Work out the finished part from the listing and answer in its coordinate system (mm). Round coordinates to 2 decimals unless told otherwise and drop trailing zeros. Write each loop counter-clockwise with the first axis right and the second up, starting at its lowest first coordinate (ties: lowest second). Pieces come first, ordered by that corner, then holes. Notation, with made-up numbers: M -33,58 L -20,58 A19 cw -20,62 Z; hole C 59.25,39 d3. An arc over 180 degrees is marked long. One line per item, written item: value. Start each with the question number.
Q1. Find section A-A (y = -73.5). Write down the section's boundary in (x, z).
Q2. Find section D-D (y = 1). Write down the section's boundary in (x, z), and give its area (3 significant figures).
Q3. Find section C-C (z = 2.4). Write down the section's boundary in (x, y).
Q4. Consider probe 1 along Y at (x, z) = (0, 1.05); probe 2 along Y at (x, z) = (-1.5, 2.65); probe 3 along X at (y, z) = (-76, 1.15). Determine where each line is inside the solid, lowest interval first.
Q5. Find section B-B (x = 0). Write down the section's boundary in (y, z).
Q6. Given pin 1 Ø4 at (x, y) = (7.5, -20.5) entering from -Z, flat-ended and moving along its own axis, determine where the tip first touches the part or whether it passes through.
from build123d import *

# Parameters (mm, degrees)
SKETCH1_R           = 2.5
BOSS_EXTRUDE1_DEPTH = 3


with BuildPart() as part:
    # Sketch1 → Boss-Extrude1 (new body)
    with BuildSketch(Plane.XY):
        with BuildLine():
            Line((10, 0), (10, -100))
            Line((10, -100), (-10, -100))
            Line((-10, -100), (-10, 0))
            ThreePointArc((-10, 0), (0, 10), (10, 0))
        make_face()
        Circle(SKETCH1_R, mode=Mode.SUBTRACT)
        with BuildLine():
            Line((5, -20), (5, -40))
            ThreePointArc((5, -40), (0, -45), (-5, -40))
            Line((-5, -40), (-5, -20))
            ThreePointArc((-5, -20), (0, -15), (5, -20))
        make_face(mode=Mode.SUBTRACT)
        with BuildLine():
            Line((-5, -85), (-5, -65))
            ThreePointArc((-5, -65), (0, -60), (5, -65))
            Line((5, -65), (5, -85))
            ThreePointArc((5, -85), (0, -90), (-5, -85))
        make_face(mode=Mode.SUBTRACT)
    extrude(amount=BOSS_EXTRUDE1_DEPTH)


solid = part.part
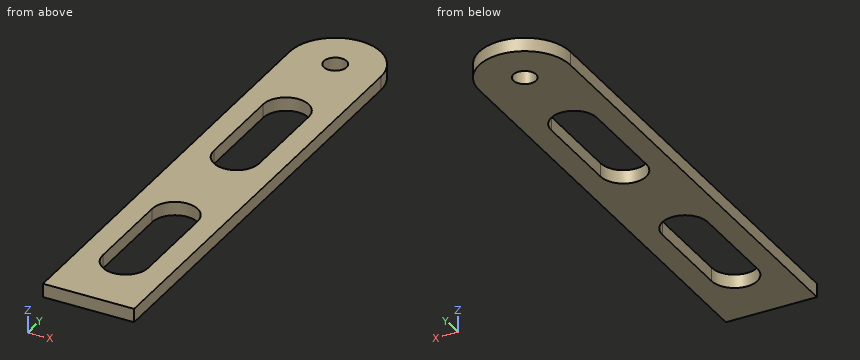
The answers:
1. outline: M -10,0 L -5,0 L -5,3 L -10,3 Z; M 5,0 L 10,0 L 10,3 L 5,3 Z
2. outline: M -9.95,0 L -2.29,0 L -2.29,3 L -9.95,3 Z; M 2.29,0 L 9.95,0 L 9.95,3 L 2.29,3 Z
2. area: 46.0 mm2
3. outline: M -10,-100 L 10,-100 L 10,0 A10 ccw -10,0 Z; hole M -5,-85 A5 ccw 5,-85 L 5,-65 A5 ccw -5,-65 Z; hole M -5,-40 A5 ccw 5,-40 L 5,-20 A5 ccw -5,-20 Z; hole C 0,0 d5
4. probe 1: -100 to -90, -60 to -45, -15 to -2.5, 2.5 to 10
4. probe 2: -100 to -89.77, -60.23 to -44.77, -15.23 to -2, 2 to 9.89
4. probe 3: -10 to -5, 5 to 10
5. outline: M -100,0 L -90,0 L -90,3 L -100,3 Z; M -60,0 L -45,0 L -45,3 L -60,3 Z; M -15,0 L -2.5,0 L -2.5,3 L -15,3 Z; M 2.5,0 L 10,0 L 10,3 L 2.5,3 Z
6. pin 1: z = 0
